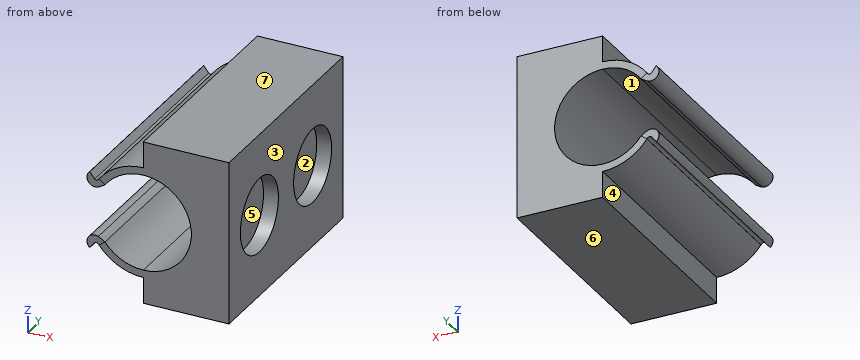
Autodesk Inventor part; units mm, degrees
ref_plane "YZ Plane" through (0, 0, 0) normal (1, 0, 0) x (0, 1, 0)
ref_plane "XZ Plane" through (0, 0, 0) normal (0, 1, 0) x (-1, 0, 0)
ref_plane "XY Plane" through (0, 0, 0) normal (0, 0, 1) x (1, 0, 0)
sketch "Эскиз1" plane through (0, 0, 0) normal (0, 1, 0) x (-1, 0, 0)
  circle A0 centre (0, 0) radius 6.45
  circle A1 centre (0, 0) radius 7.45
  line L0 (0, 0) -> (5.9449, 4.49)
  line L1 (0, 0) -> (5.9449, -4.49)
  point P0 (5.147, -3.8873)
  point P1 (5.147, 3.8873)
  dimension "d0" = 12.9
  dimension "d1" = 14.9
extrude "Выдавливание1" add sketch "Эскиз1" along normal blind 30 contours A0 L1 A1 L0 picked at (-6.4749, 2.8302)
sketch "Эскиз2" plane through (0, 30, 0) normal (0, 1, 0) x (1, 0, 0)
  arc A0 (-5.147, -3.8873) -> (-6.0397, -3.3574) centre (-7.8483, -7.4212) ccw
  arc A1 (-6.0397, -3.3574) -> (-7.1966, -5.1632) centre (-6.474, -4.3526) ccw
  line L0 (-7.1966, -5.1632) -> (-6.5253, -4.3087)
  arc A2 (-5.9464, -4.4755) -> (-6.5253, -4.3087) centre (-6.3147, -4.6659) ccw
  line L1 (-5.147, -3.8873) -> (-5.9449, -4.49)
  line L2 (-5.9449, -4.49) -> (-5.147, -3.8873)
  line L3 (-5.9449, -4.49) -> (-5.9464, -4.4755)
  line L4 (-0.0151, 0) -> (-3.489, 0)
  arc A3 (-6.0397, 3.3574) -> (-5.147, 3.8873) centre (-7.8483, 7.4212) ccw
  arc A4 (-6.5253, 4.3087) -> (-5.9464, 4.4755) centre (-6.3147, 4.6659) ccw
  line L5 (-5.147, 3.8873) -> (-5.9449, 4.49)
  line L6 (-5.9449, 4.49) -> (-5.147, 3.8873)
  line L7 (-5.9449, 4.49) -> (-5.9464, 4.4755)
  arc A5 (-7.1966, 5.1632) -> (-6.0397, 3.3574) centre (-6.474, 4.3526) ccw
  line L8 (-7.1966, 5.1632) -> (-6.5253, 4.3087)
  point P0 (-5.147, 3.8873)
  point P1 (-5.9449, -4.49)
  point P2 (-5.3694, -4.0591)
  point P3 (-5.9449, 4.49)
  point P4 (-5.3694, 4.0591)
  point P5 (-5.9449, 4.49)
  dimension "d25" = 1.0859
sketch "Эскиз3" plane through (0, 30, 0) normal (0, 1, 0) x (1, 0, 0)
  arc A0 (-5.9449, -4.49) -> (-5.9449, 4.49) centre (0, 0) ccw
  line L0 (11.5, -6.95) -> (11.5, 6.95)
  arc A1 (-5.147, -3.8873) -> (-5.147, 3.8873) centre (0, 0) ccw
  line L1 (0, -7.45) -> (0, -6.45)
  line L2 (0, 6.45) -> (0, 7.45)
  line L3 (11.5, 6.95) -> (11.5, 10.95)
  line L4 (11.5, -6.95) -> (11.5, -10.95)
  line L5 (0, 2.95) -> (0, 7.45)
  line L6 (11.5, -10.95) -> (0, -10.95)
  line L7 (0, -10.95) -> (0, -7.45)
  line L8 (11.5, 10.95) -> (0, 10.95)
  line L9 (0, 10.95) -> (0, 7.45)
  arc A2 (0, -6.45) -> (0, 6.45) centre (0, 0) ccw
  dimension "d13" = 4
  dimension "d14" = 4
  dimension "d22" = 21.9
  dimension "d23" = 4.5
extrude "Выдавливание3" add sketch "Эскиз3" against normal blind 30
ref_plane "РабПлоскость1" through (11.5, 20, 4.95) normal (1, 0, 0) x (0, 0, -1)
sketch "Эскиз4" plane through (11.5, 20, 4.95) normal (1, 0, 0) x (0, 0, -1)
  line L0 (4.95, -20) -> (4.95, 10)
  line L1 (1, 10) -> (8.9, 10)
  circle A0 centre (4.95, -12) radius 5
  line L2 (14.4, -20) -> (-4.5, -20)
  circle A1 centre (4.95, 2) radius 5
  line L3 (-4.5, 10) -> (14.4, 10)
  point P0 (7.3306, 10)
  point P1 (2.5694, 10)
  point P2 (4.95, 10)
  dimension "d15" = 10
  dimension "d16" = 8
  dimension "d17" = 10
  dimension "d18" = 8
extrude "Выдавливание4" cut sketch "Эскиз4" against normal blind 2
extrude "Выдавливание5" add sketch "Эскиз2" against normal blind 30
sketch "Эскиз5" plane through (0, 30, 0) normal (0, 1, 0) x (1, 0, 0)
  arc A0 (0, 7.45) -> (-5.9449, 4.49) centre (0, 0) ccw
  line L0 (-5.9449, 4.49) -> (-5.9464, 4.4755)
  arc A1 (-6.5253, 4.3087) -> (-5.9464, 4.4755) centre (-6.3147, 4.6659) ccw
  line L1 (-6.5253, 4.3087) -> (-7.1966, 5.1632)
  arc A2 (-7.1966, 5.1632) -> (-6.0397, 3.3574) centre (-6.474, 4.3526) ccw
  arc A3 (-6.0397, 3.3574) -> (-5.147, 3.8873) centre (-7.8483, 7.4212) ccw
  arc A4 (-5.147, -3.8873) -> (-5.147, 3.8873) centre (0, 0) ccw
  arc A5 (-5.147, -3.8873) -> (-6.0397, -3.3574) centre (-7.8483, -7.4212) ccw
  arc A6 (-6.0397, -3.3574) -> (-7.1966, -5.1632) centre (-6.474, -4.3526) ccw
  line L2 (-7.1966, -5.1632) -> (-6.5253, -4.3087)
  arc A7 (-5.9464, -4.4755) -> (-6.5253, -4.3087) centre (-6.3147, -4.6659) ccw
  line L3 (-5.9464, -4.4755) -> (-5.9449, -4.49)
  arc A8 (-5.9449, -4.49) -> (0, -7.45) centre (0, 0) ccw
  line L4 (0, -7.45) -> (0, -10.95)
  line L5 (0, -10.95) -> (11.5, -10.95)
  line L6 (11.5, -10.95) -> (11.5, 10.95)
  line L7 (11.5, 10.95) -> (0, 10.95)
  line L8 (0, 10.95) -> (0, 7.45)
  line L9 (0, 6.45) -> (0, 7.45)
  line L10 (0, -6.45) -> (0, -7.45)
sketch "Эскиз6" plane through (11.5, 30, 10.95) normal (1, 0, 0) x (0, 0, -1)
  arc A0 (15.95, -22) -> (15.95, -22) centre (10.95, -22) ccw
  arc A1 (15.95, -8) -> (15.95, -8) centre (10.95, -8) ccw
  point P0 (10.95, -30)
properties part number "крепление маркера 13мм"
Check sheet for the modelled part. Datum: model origin and axes. Units: mm. Face numbers are marked on the shaded views. A direction names the side the tool comes from. Coordinates: 2 decimals unless noted, no trailing zeros. Order: outer loops, then holes, each group sorted by start corner. A loop starts at its lowest first (then second) coordinate and runs counter-clockwise, first axis right, second up. Notation, with made-up numbers: (-3, 63.25) -> (45, 63.25) arc R7 ccw to (45, 72.25) -> close; hole circle Ø1 at (-3.75, 33). An arc over 180 degrees is marked (long way). Write item = value, one per line. Start each with the question number.
1) Cross-section at D-D (x = 5). Enter the section's corners in (y, z), then the cut area to 3 significant figures.
2) Go/stop test with flat-tipped pins: P1, Ø1.7, axis at y = 22, z = -10, coming from the -X side; P2, Ø4, axis at x = -4, y = 17.5, coming from the +Z side; P3, Ø8, axis at y = 22, z = 0, coming from the +X side. Record where each tip stops, or that it passes through.
3) Cross-section at A-A (x = -1.5). Enter the section's corners in (y, z).
4) Access from +Z, -Z, +X, -X, +Y, -Y to the whole of each face (thin tool, end or side, straight path). Record for the marked faces 1, 2, 3 and 4.
5) Material ranges on L1, parallel to Y at x = 11, z = 0; L2, parallel to Z at x = 10.65, y = 8; L3, parallel to X at y = 25.25, z = 9.5, recorded low to high.
6) Mould release check, pull along Z, two halves, no side actions. Record for the marked faces 5, 6 and 7: +Z half, -Z half, draft (parallel to the pull), parting line (faces both ways), or undercut.
7) Cross-section at B-B (z = 0). Enter the section's corners in (x, y), then the cut area to 3 significant figures.
Ans:
q1.outline = (0, -10.95) -> (30, -10.95) -> (30, -4.07) -> (0, -4.07) -> close; (0, 4.07) -> (30, 4.07) -> (30, 10.95) -> (0, 10.95) -> close
q1.area = 413 mm²
q2.P1 = 0
q2.P2 = 7.18
q2.P3 = 9.5
q3.outline = (0, -7.3) -> (30, -7.3) -> (30, -6.27) -> (0, -6.27) -> close; (0, 6.27) -> (30, 6.27) -> (30, 7.3) -> (0, 7.3) -> close
q4.face_1 = +Y, -Y
q4.face_2 = +X
q4.face_3 = +Z, -Z, +X, +Y, -Y
q4.face_4 = -Z, -X, +Y, -Y
q5.L1 = 0 to 3, 13 to 17, 27 to 30
q5.L2 = -10.95 to -5, 5 to 10.95
q5.L3 = 0 to 11.5
q6.face_5 = undercut
q6.face_6 = -Z half
q6.face_7 = +Z half
q7.outline = (6.45, 0) -> (11.5, 0) -> (11.5, 3) -> (9.5, 3) -> (9.5, 13) -> (11.5, 13) -> (11.5, 17) -> (9.5, 17) -> (9.5, 27) -> (11.5, 27) -> (11.5, 30) -> (6.45, 30) -> close
q7.area = 111 mm²
